Read the model definition and answer for the solid it produces. Units are mm, in the model's axes. A direction names the side the tool comes from. Round coordinates to 2 decimals unless told otherwise and drop trailing zeros. Write each loop counter-clockwise with the first axis right and the second up, starting at its lowest first coordinate (ties: lowest second). Pieces come first, ordered by that corner, then holes. Notation, with made-up numbers: (53.5, 66) -> (89.5, 66) arc R11 ccw to (89.5, 74) -> close; hole circle Ø6 at (-18, 68). An arc over 180 degrees is marked (long way). Return JSON: item names as keys, results as strings.
from build123d import *

# Parameters (mm, degrees)
SKICA1_W                 = 54.6
SKICA1_H                 = 54.6
P_IDAT_VYSUNUT_M2_DEPTH  = 3
SKICA5_W                 = 54.6
SKICA5_H                 = 5
ODEBRAT_VYSUNUT_M3_DEPTH = 1
SKICA14_W                = 52.6
SKICA14_H                = 1
P_IDAT_VYSUNUT_M9_DEPTH  = 15
SKICA17_R                = 2
ODEBRAT_VYSUNUT_M8_DEPTH = 4
SKICA19_W                = 7.8
SKICA19_H                = 7.8
P_IDAT_VYSUNUT_M10_DEPTH = 18
SKICA20_R                = 2.4
ODEBRAT_VYSUNUT_M9_DEPTH = 1.7
ZAOBLIT1_R               = 3


with BuildPart() as part:
    # Skica1 → Přidat vysunutím2 (new body)
    with BuildSketch(Plane.XY):
        Rectangle(SKICA1_W, SKICA1_H)
    extrude(amount=P_IDAT_VYSUNUT_M2_DEPTH)

    # Skica5 → Odebrat vysunutím3 (cut)
    with BuildSketch(Plane(origin=(0, 0, 0), x_dir=(-1, 0, 0), z_dir=(0, 0, -1))):
        Rectangle(SKICA5_W, SKICA5_H)
    extrude(amount=-ODEBRAT_VYSUNUT_M3_DEPTH, mode=Mode.SUBTRACT)

    # Skica14 → Přidat vysunutím9 (add)
    with BuildSketch(Plane.XY.offset(3)):
        Polygon((27.3, 27.3), (-27.3, 27.3), (-27.3, -27.3), (-26.3, -27.3), (-26.3, -26.3), (-26.3, 26.3), (26.3, 26.3), (26.3, -26.3), (26.3, -27.3), (27.3, -27.3), align=None)
        with Locations((0, -26.8)):
            Rectangle(SKICA14_W, SKICA14_H)
    extrude(amount=P_IDAT_VYSUNUT_M9_DEPTH)

    # Skica17 → Odebrat vysunutím8 (cut)
    with BuildSketch(Plane(origin=(0, 0, 1), x_dir=(-1, 0, 0), z_dir=(0, 0, -1))):
        with Locations((-20.3, 0)):
            Circle(SKICA17_R)
        with Locations((20.3, 0)):
            Circle(SKICA17_R)
    extrude(amount=-ODEBRAT_VYSUNUT_M8_DEPTH, mode=Mode.SUBTRACT)

    # Skica19 → Přidat vysunutím10 (add)
    with BuildSketch(Plane(origin=(0, 0, 0), x_dir=(-1, 0, 0), z_dir=(0, 0, -1))):
        with Locations((-23.4, 23.4)):
            Rectangle(SKICA19_W, SKICA19_H)
        with Locations((23.4, 23.4)):
            Rectangle(SKICA19_W, SKICA19_H)
        with Locations((-23.4, -23.4)):
            Rectangle(SKICA19_W, SKICA19_H)
        with Locations((23.4, -23.4)):
            Rectangle(SKICA19_W, SKICA19_H)
    extrude(amount=-P_IDAT_VYSUNUT_M10_DEPTH)

    # Skica20 → Odebrat vysunutím9 (cut)
    with BuildSketch(Plane.XY.offset(18)):
        with Locations((-23.4, -23.4)):
            Circle(SKICA20_R)
        with Locations((-23.4, 23.4)):
            Circle(SKICA20_R)
        with Locations((23.400280565, 23.4)):
            Circle(SKICA20_R)
        with Locations((23.400280565, -23.4)):
            Circle(SKICA20_R)
    extrude(amount=-ODEBRAT_VYSUNUT_M9_DEPTH, mode=Mode.SUBTRACT)

    # Zaoblit1
    zaoblit1_edges = [part.edges().sort_by_distance(p)[0] for p in [
        (19.5, -19.5, 10.5),
        (-19.5, -19.5, 10.5),
        (19.5, 19.5, 10.5),
        (-19.5, 19.5, 10.5),
    ]]
    fillet(zaoblit1_edges, radius=ZAOBLIT1_R)


solid = part.part
Item 1: A tool of negligible diameter and unlimited length cuts with its end or side. For faces 3 (the cylindrical face through (-18.302, 0.088, 1.986)), 4 (the flat face through (23, -23, 16.3)), from which of +Z, -Z, +X, -X, +Y, -Y can it reach the whole face along a straight path? Write none if from no direction.
Worked answers:
{"face 3": "+Z, -Z", "face 4": "+Z"}
Item 2: Section A-A (y = 0) is taken. Give the vertices of the cut face in (x, z), then the cut area to 3 significant figures.
Worked answers:
{"outline": "(-27.3, 1) -> (-22.3, 1) -> (-22.3, 3) -> (-26.3, 3) -> (-26.3, 18) -> (-27.3, 18) -> close; (-18.3, 1) -> (18.3, 1) -> (18.3, 3) -> (-18.3, 3) -> close; (22.3, 1) -> (27.3, 1) -> (27.3, 18) -> (26.3, 18) -> (26.3, 3) -> (22.3, 3) -> close", "area": "123 mm2"}
Item 3: Section B-B (z = 12.5) is taken. Give the vertices of the cut face in (x, y), then the cut area to 3 significant figures.
Worked answers:
{"outline": "(-27.3, -27.3) -> (27.3, -27.3) -> (27.3, 27.3) -> (-27.3, 27.3) -> close; hole (-26.3, -19.5) -> (-22.5, -19.5) arc R3 cw to (-19.5, -22.5) -> (-19.5, -26.3) -> (19.5, -26.3) -> (19.5, -22.5) arc R3 cw to (22.5, -19.5) -> (26.3, -19.5) -> (26.3, 19.5) -> (22.5, 19.5) arc R3 cw to (19.5, 22.5) -> (19.5, 26.3) -> (-19.5, 26.3) -> (-19.5, 22.5) arc R3 cw to (-22.5, 19.5) -> (-26.3, 19.5) -> close", "area": "392 mm2"}
Item 4: Section D-D (y = 11) is taken. Give the vertices of the cut face in (x, z), then the cut area to 3 significant figures.
Worked answers:
{"outline": "(-27.3, 0) -> (27.3, 0) -> (27.3, 18) -> (26.3, 18) -> (26.3, 3) -> (-26.3, 3) -> (-26.3, 18) -> (-27.3, 18) -> close", "area": "194 mm2"}
Item 5: Section C-C (x = -23.4) is taken. Give the vertices of the cut face in (y, z), then the cut area to 3 significant figures.
Worked answers:
{"outline": "(-27.3, 0) -> (-2.5, 0) -> (-2.5, 1) -> (2.5, 1) -> (2.5, 0) -> (27.3, 0) -> (27.3, 18) -> (25.8, 18) -> (25.8, 16.3) -> (21, 16.3) -> (21, 18) -> (19.5, 18) -> (19.5, 3) -> (-19.5, 3) -> (-19.5, 18) -> (-21, 18) -> (-21, 16.3) -> (-25.8, 16.3) -> (-25.8, 18) -> (-27.3, 18) -> close", "area": "376 mm2"}
Item 6: Flat-ended cylindrical pins translate along their axes: pin 1 (3 mm diameter, centred on x = 7.5, y = -19, fed in from +Z); pin 2 (1.4 mm diameter, centred on x = -23, y = 23, fed in from +Z). Find the tip coordinate at first contact, or state that the pin passes through.
Worked answers:
{"pin 1": "stops at z = 3", "pin 2": "stops at z = 16.3"}
Item 7: Straight lines are drawn through the part: L1, parallel to Y at x = -23.4, z = 17.45; L2, parallel to Y at x = 20.5, z = 1.25; L3, parallel to Y at x = 10, z = 10.75. For each, find the intervals that lie inside material, in ascending order. Write a range as [from, to].
Worked answers:
{"L1": "y = [-27.3, -25.8], [-21, -19.5], [19.5, 21], [25.8, 27.3]", "L2": "y = [-27.3, -1.99], [1.99, 27.3]", "L3": "y = [-27.3, -26.3], [26.3, 27.3]"}
Item 8: For a pull along X with two mould halves and no side action, classify faces 1 (the flat face through (-23, 23, 16.3)), 2 (the flat face through (-27.3, 0, 9)) as released by +X, released by -X, zero draft, split by the parting line, or undercut.
Worked answers:
{"face 1": "undercut", "face 2": "released by -X"}
